from build123d import *

# Parameters (mm, degrees)
SKETCH1_W              = 165.1
SKETCH1_H              = 95.25
BOSS_EXTRUDE1_DEPTH    = 1.27
SKETCH2_W              = 1.27
SKETCH2_H              = 95.25
BOSS_EXTRUDE2_DEPTH    = 19.05
CONVERT_SOLID1_START   = 35.497339992
CONVERT_SOLID1_DEPTH   = 95.25
CONVERT_SOLID1_2_DEPTH = 95.25
SKETCH7_R              = 1.7272
CUT_EXTRUDE1_DEPTH     = 215.065982678
SKETCH8_R              = 1.7526
CUT_EXTRUDE2_DEPTH     = 212.461058862


# Read off the part's stored shape, not the designer's step: Convert-Solid1
with BuildPart() as part:
    # Sketch1 → Boss-Extrude1 (new body)
    with BuildSketch(Plane.XY):
        with Locations((-85.725, 83.122339992)):
            Rectangle(SKETCH1_W, SKETCH1_H)
    extrude(amount=BOSS_EXTRUDE1_DEPTH)

    # Sketch2 → Boss-Extrude2 (add)
    with BuildSketch(Plane(origin=(0, 0, 0), x_dir=(-1, 0, 0), z_dir=(0, 0, -1))):
        with Locations((3.81, 83.122339992)):
            Rectangle(SKETCH2_W, SKETCH2_H)
        with Locations((167.64, 83.122339992)):
            Rectangle(SKETCH2_W, SKETCH2_H)
    extrude(amount=BOSS_EXTRUDE2_DEPTH)

    # Convert-Solid1 outline → Convert-Solid1 (cut)
    with BuildSketch(Plane(origin=(0, 0, 0), x_dir=(1, 0, 0), z_dir=(0, 1, 0)).offset(CONVERT_SOLID1_START)):
        with BuildLine():
            ThreePointArc((-3.175, 1.27), (-3.918948776, -0.526051224), (-5.715, -1.27))
            Line((-5.715, -1.27), (-3.175, -1.27))
            Line((-3.175, -1.27), (-3.175, 1.27))
        make_face()
        with BuildLine():
            ThreePointArc((-165.735, -1.27), (-167.531051224, -0.526051224), (-168.275, 1.27))
            Line((-168.275, 1.27), (-168.275, -1.27))
            Line((-168.275, -1.27), (-165.735, -1.27))
        make_face()
    extrude(amount=CONVERT_SOLID1_DEPTH, mode=Mode.SUBTRACT)

    # Convert-Solid1 2 outline → Convert-Solid1 2 (add)
    with BuildSketch(Plane(origin=(0, 0, 0), x_dir=(1, 0, 0), z_dir=(0, 1, 0)).offset(CONVERT_SOLID1_START)):
        with BuildLine():
            ThreePointArc((-4.445, 1.27), (-4.816974388, 0.371974388), (-5.715, 0))
            Line((-5.715, 0), (-4.445, 0))
            Line((-4.445, 0), (-4.445, 1.27))
        make_face()
        with BuildLine():
            ThreePointArc((-165.735, 0), (-166.633025612, 0.371974388), (-167.005, 1.27))
            Line((-167.005, 1.27), (-167.005, 0))
            Line((-167.005, 0), (-165.735, 0))
        make_face()
    extrude(amount=CONVERT_SOLID1_2_DEPTH)

    # Sketch7 → Cut-Extrude1 (cut, through all)
    with BuildSketch(Plane.XY.offset(1.27)):
        with Locations((-7.8232, 109.792339992)):
            Circle(SKETCH7_R)
        with Locations((-48.1584, 109.792339992)):
            Circle(SKETCH7_R)
        with Locations((-88.4936, 109.792339992)):
            Circle(SKETCH7_R)
        with Locations((-128.8288, 109.792339992)):
            Circle(SKETCH7_R)
        with Locations((-163.83, 54.547339992)):
            Circle(SKETCH7_R)
        with Locations((-123.4948, 54.547339992)):
            Circle(SKETCH7_R)
        with Locations((-83.1596, 54.547339992)):
            Circle(SKETCH7_R)
        with Locations((-42.8244, 54.547339992)):
            Circle(SKETCH7_R)
    extrude(amount=-CUT_EXTRUDE1_DEPTH, mode=Mode.SUBTRACT)

    # Sketch8 → Cut-Extrude2 (cut, through all)
    with BuildSketch(Plane.ZY.offset(168.275)):
        with Locations((-11.43, 40.577339992)):
            Circle(SKETCH8_R)
        with Locations((-11.43, 124.397339992)):
            Circle(SKETCH8_R)
    extrude(amount=-CUT_EXTRUDE2_DEPTH, mode=Mode.SUBTRACT)


solid = part.part
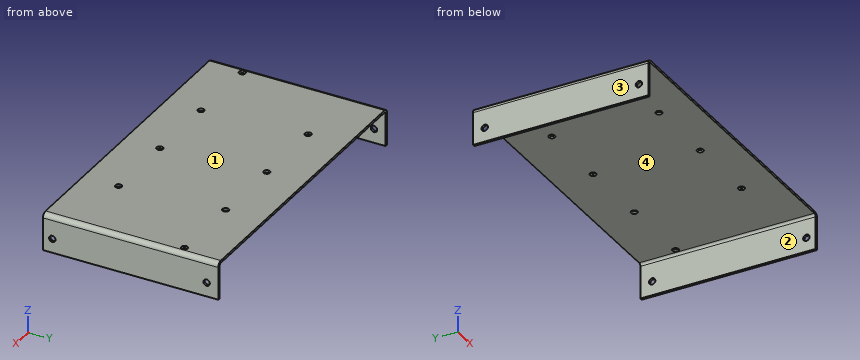
Geometry check sheet. Reference: the model listing, model coordinates, mm. Face numbers are marked on the shaded views. Coordinates: 2 decimals unless noted, no trailing zeros. Order: outer loops, then holes, each group sorted by start corner. A loop starts at its lowest first (then second) coordinate and runs counter-clockwise, first axis right, second up. Notation, with made-up numbers: (-14.75, -28) -> (12.25, -28) arc R27 ccw to (12.25, 10) -> close; hole circle Ø6 at (57.5, 37.5). An arc over 180 degrees is marked (long way). Use a Markdown table: item, result. Add a question column.
1. Go/stop test with a flat-tipped pin: pin 1 Ø4.5 at (x, y) = (-42.82, 54.55) entering from -Z. Record where the tip stops, or that it passes through.
2. Cross-section at B-B (x = -163.83). Enter the section's corners in (y, z).
3. Cross-section at D-D (x = -83). Enter the section's corners in (y, z).
4. Mould release check, pull along X, two halves, no side actions. Record for the marked faces 1, 2, 3 and 4: pulls with the +X half, pulls with the -X half, needs draft (parallel to the pull), parting line crosses it, or undercut.
5. Cross-section at C-C (y = 80). Enter the section's corners in (x, z) (3 decimals), and give its area (3 significant figures).
6. Cross-section at A-A (z = -11.43). Enter the section's corners in (x, y) (3 decimals).
7. Material ranges on L1, parallel to Y at x = -3.6, z = -11.43; L2, parallel to Y at x = -163.83, z = 0.8; L3, parallel to X at y = 85, z = -17.5 (3 decimals), recorded low to high.
Filled sheet:
| question | item | result |
|---|---|---|
| 1 | pin 1 | z = 0 |
| 2 | outline | (35.5, 0) -> (52.82, 0) -> (52.82, 1.27) -> (35.5, 1.27) -> close; (56.27, 0) -> (130.75, 0) -> (130.75, 1.27) -> (56.27, 1.27) -> close |
| 3 | outline | (35.5, 0) -> (52.83, 0) -> (52.83, 1.27) -> (35.5, 1.27) -> close; (56.27, 0) -> (130.75, 0) -> (130.75, 1.27) -> (56.27, 1.27) -> close |
| 4 | face 1 | needs draft |
| 4 | face 2 | undercut |
| 4 | face 3 | pulls with the -X half |
| 4 | face 4 | undercut |
| 5 | outline | (-168.275, -19.05) -> (-167.005, -19.05) -> (-167.005, -1.27) arc R1.27 cw to (-165.735, 0) -> (-5.715, 0) arc R1.27 cw to (-4.445, -1.27) -> (-4.445, -19.05) -> (-3.175, -19.05) -> (-3.175, -1.27) arc R2.54 ccw to (-5.715, 1.27) -> (-165.735, 1.27) arc R2.54 ccw to (-168.275, -1.27) -> close |
| 5 | area | 256 mm2 |
| 6 | outline | (-168.275, 35.497) -> (-167.005, 35.497) -> (-167.005, 38.825) -> (-168.275, 38.825) -> close; (-168.275, 42.33) -> (-167.005, 42.33) -> (-167.005, 122.645) -> (-168.275, 122.645) -> close; (-168.275, 126.15) -> (-167.005, 126.15) -> (-167.005, 130.747) -> (-168.275, 130.747) -> close; (-4.445, 35.497) -> (-3.175, 35.497) -> (-3.175, 38.825) -> (-4.445, 38.825) -> close; (-4.445, 42.33) -> (-3.175, 42.33) -> (-3.175, 122.645) -> (-4.445, 122.645) -> close; (-4.445, 126.15) -> (-3.175, 126.15) -> (-3.175, 130.747) -> (-4.445, 130.747) -> close |
| 7 | L1 | 35.5 to 38.82, 42.33 to 122.64, 126.15 to 130.75 |
| 7 | L2 | 35.5 to 52.82, 56.27 to 130.75 |
| 7 | L3 | -168.275 to -167.005, -4.445 to -3.175 |
